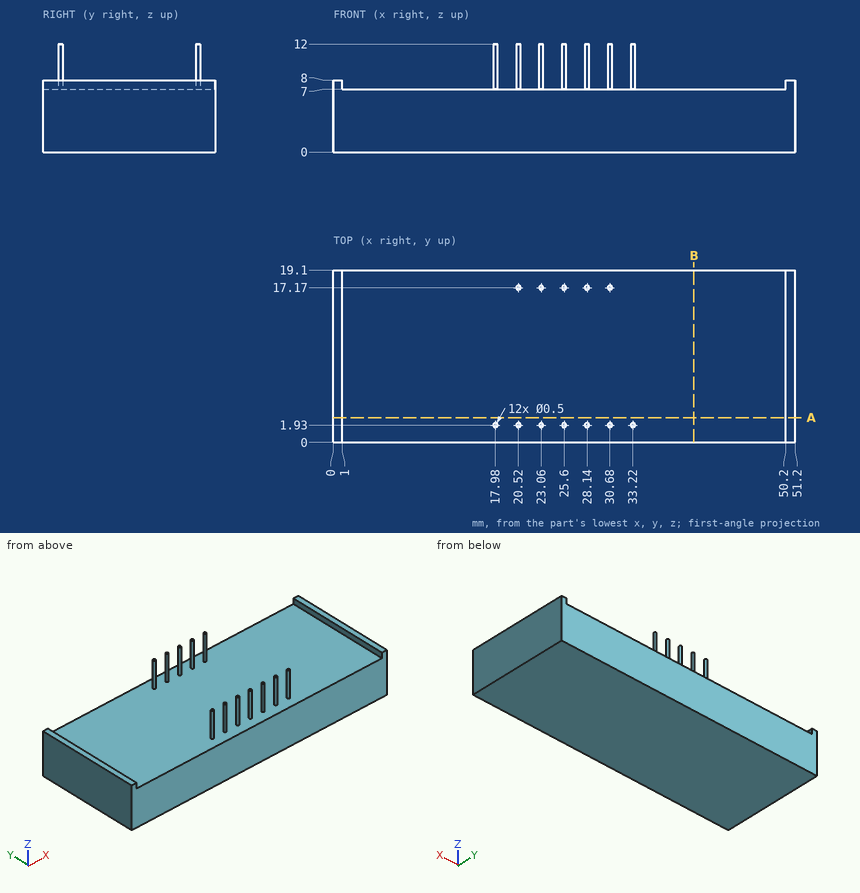
Could you check a few things on this drawing? It's one solid part, dimensions in mm from its lowest x, y, z. Round coordinates to 2 decimals unless told otherwise and drop trailing zeros. Loops run counter-clockwise (first coordinate to the right, second up) from the corner with the lowest first, then second, coordinate; pieces in that order, holes last.
Q1. I want a section at B-B (x = 40). Write out the boundary of the cut face in (y, z).
Q2. Please list where these lines run through material, in increasing order: L1, parallel to X at y = 11.75, z = 7.5; L2, parallel to Z at x = 31, y = 4.5.
Q3. I want a section at A-A (y = 2.75). Write out the boundary of the cut face in (x, z).
Q4. For P1, Ø3, axis at x = 17.5, y = 16.5, coming from the +Z side; P2, Ø1.1, axis at x = 51, y = 9, coming from the +Z side, each with a flat end and sliding along its axis, tell me the tip position at first contact or that it passes through.
Answer below:
1. outline: (0, 0) - (19.1, 0) - (19.1, 7) - (0, 7) - close
2. L1: x = 0 to 1, 50.2 to 51.2
2. L2: z = 0 to 7
3. outline: (0, 0) - (51.2, 0) - (51.2, 8) - (50.2, 8) - (50.2, 7) - (1, 7) - (1, 8) - (0, 8) - close
4. P1: stops at z = 7
4. P2: stops at z = 8
